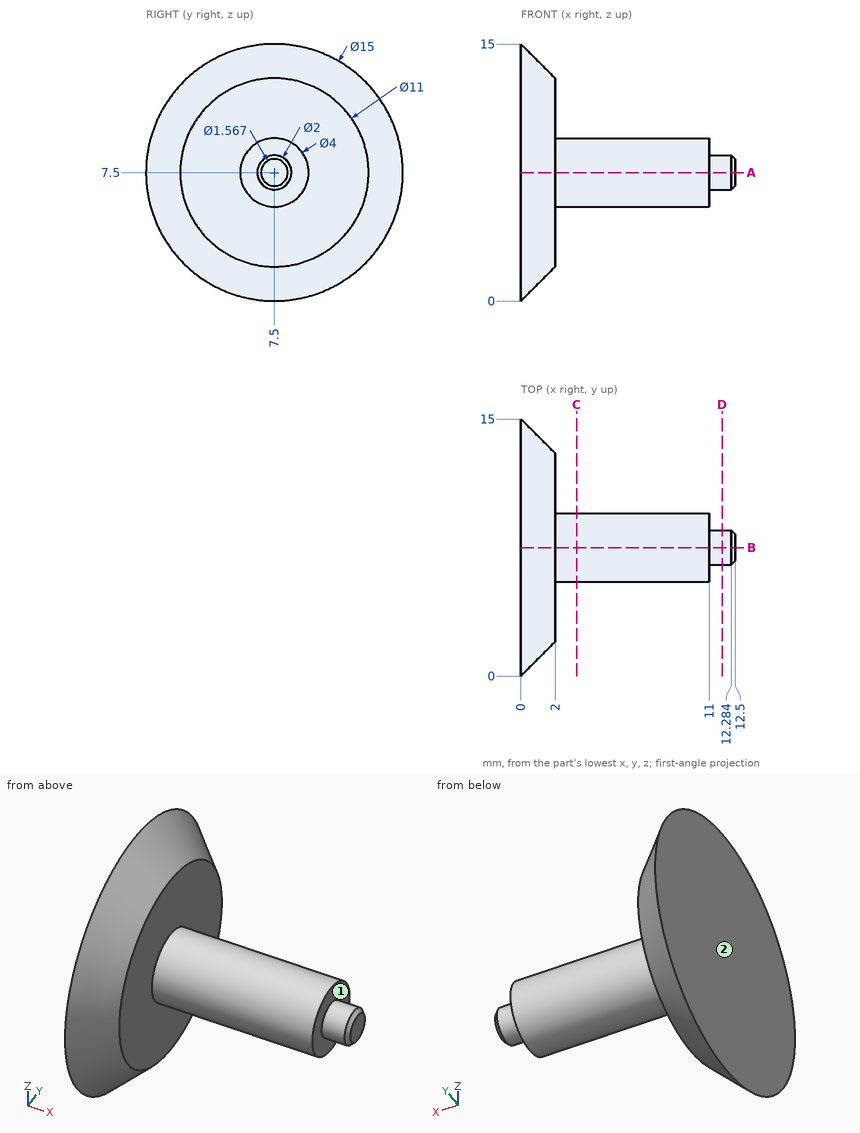
Can you work these out from the drawing? Everything is in mm from the part's minimum corner. A direction names the side the tool comes from. Give positions to 0.01 mm unless a question says otherwise; leave off trailing zeros. Order: outer loops, then holes, each group sorted by start corner. A loop starts at its lowest first (then second) coordinate and runs counter-clockwise, first axis right, second up.
1. Will these pins go through, and if not, where does the flat tip stop? P1, Ø8, axis at y = 11.5, z = 3, coming from the -X side; P2, Ø4, axis at x = 10, y = 12.5, coming from the -Z side.
2. Suppose I cut it at C-C (x = 3.25). List the corners of the cut face in (y, z) for me, plus the area to 3 significant figures.
3. For the marked faces 1 and 2, which set-ups out of +Z, -Z, +X, -X, +Y, -Y let a thin tool reach every point of the face, with its end or its side?
4. I need wall thicknesses on L1, parallel to X at y = 12.75, z = 6.5; L2, parallel to Y at x = 2.5, z = 7.5; L3, parallel to Z at x = 4.25, y = 8.25 (1 decimal). Which ranges of each line are inside material? Lowest first, please.
5. Suppose I cut it at D-D (x = 11.75). List the corners of the cut face in (y, z) for me.
6. Suppose I cut it at A-A (z = 7.5). List the corners of the cut face in (x, y) for me.
Solved:
1. P1: stops at x = 0
1. P2: passes through
2. outline: circle Ø4 at (7.5, 7.5)
2. area: 12.6 mm2
3. face 1: +X
3. face 2: +Z, -Z, -X, +Y, -Y
4. L1: x = 0 to 2
4. L2: y = 5.5 to 9.5
4. L3: z = 5.6 to 9.4
5. outline: circle Ø2 at (7.5, 7.5)
6. outline: (0, 0) - (2, 2) - (2, 5.5) - (11, 5.5) - (11, 6.5) - (12.28, 6.5) - (12.5, 6.72) - (12.5, 8.28) - (12.28, 8.5) - (11, 8.5) - (11, 9.5) - (2, 9.5) - (2, 13) - (0, 15) - close
